from build123d import *

# Parameters (mm, degrees)
BOSS_EXTRUDE1_DEPTH = 14.2875
SKETCH2_R           = 5.9436
BOSS_EXTRUDE2_DEPTH = 0.9906
SKETCH3_R           = 6.35
BOSS_EXTRUDE3_DEPTH = 0.79375
CHAMFER1_SIZE       = 0.254
SKETCH4_R           = 3.175
CUT_EXTRUDE1_DEPTH  = 12.7
BOSS_EXTRUDE4_DEPTH = 43.1165
BOSS_EXTRUDE5_START = 0.9906
SKETCH6_R           = 5.9436
BOSS_EXTRUDE5_DEPTH = 0.9906
BOSS_EXTRUDE6_START = 0.79375
SKETCH7_R           = 6.35
BOSS_EXTRUDE6_DEPTH = 0.79375
CHAMFER2_SIZE       = 0.254


with BuildPart() as part:
    # Sketch1 → Boss-Extrude1 (new, symmetric)
    with BuildSketch(Plane.XY):
        Polygon((7.332348419, 0), (3.666174209, 6.35), (-3.666174209, 6.35), (-7.332348419, 0), (-3.666174209, -6.35), (3.666174209, -6.35), align=None)
    extrude(amount=BOSS_EXTRUDE1_DEPTH, both=True)

    # Sketch2 → Boss-Extrude2 (add)
    with BuildSketch(Plane(origin=(0, 0, -14.2875), x_dir=(-1, 0, 0), z_dir=(0, 0, -1))):
        with Locations(Location((0, 0, 0), (0, 0, 180))):
            Circle(SKETCH2_R)
    extrude(amount=BOSS_EXTRUDE2_DEPTH)

    # Sketch3 → Boss-Extrude3 (add)
    with BuildSketch(Plane(origin=(0, 0, -15.2781), x_dir=(-1, 0, 0), z_dir=(0, 0, -1))):
        Circle(SKETCH3_R)
    extrude(amount=BOSS_EXTRUDE3_DEPTH)

    # Chamfer1
    chamfer1_edges = [part.edges().sort_by_distance(p)[0] for p in [
        (6.35, 0, -16.07185),
    ]]
    chamfer(chamfer1_edges, length=CHAMFER1_SIZE)

    # Sketch4 → Cut-Extrude1 (cut)
    with BuildSketch(Plane(origin=(0, 0, -16.07185), x_dir=(-1, 0, 0), z_dir=(0, 0, -1))):
        Circle(SKETCH4_R)
    extrude(amount=-CUT_EXTRUDE1_DEPTH, mode=Mode.SUBTRACT)

    # Sketch5 → Boss-Extrude4 (add)
    with BuildSketch(Plane.XY.offset(14.2875)):
        Polygon((3.666174209, 6.35), (-3.666174209, 6.35), (-7.332348419, 0), (-3.666174209, -6.35), (3.666174209, -6.35), (7.332348419, 0), align=None)
    extrude(amount=BOSS_EXTRUDE4_DEPTH)

    # Sketch6 → Boss-Extrude5 (add)
    with BuildSketch(Plane.XY.offset(57.404).offset(BOSS_EXTRUDE5_START)):
        Circle(SKETCH6_R)
    extrude(amount=-BOSS_EXTRUDE5_DEPTH)

    # Sketch7 → Boss-Extrude6 (add)
    with BuildSketch(Plane.XY.offset(58.3946).offset(BOSS_EXTRUDE6_START)):
        with Locations(Location((0, 0, 0), (0, 0, 180))):
            Circle(SKETCH7_R)
    extrude(amount=-BOSS_EXTRUDE6_DEPTH)

    # Chamfer2
    chamfer2_edges = [part.edges().sort_by_distance(p)[0] for p in [
        (6.35, 0, 59.18835),
    ]]
    chamfer(chamfer2_edges, length=CHAMFER2_SIZE)


solid = part.part
Design review of the part built by this model. Coordinates are the model's own, in mm. A direction names the side the tool comes from. Round coordinates to 2 decimals unless told otherwise and drop trailing zeros. Write each loop counter-clockwise with the first axis right and the second up, starting at its lowest first coordinate (ties: lowest second). Pieces come first, ordered by that corner, then holes. Notation, with made-up numbers: (-39, 0) - (-10, 0) arc R12 ccw to (-10, 7) - close; hole circle Ø4 at (-17, 85). An arc over 180 degrees is marked (long way). Use a Markdown table: item, result. Add a question column.
1. Wall thickness on probe 1 along Y at (x, z) = (0, -11) (3 decimals); probe 2 along Z at (x, y) = (5, -3.75); probe 3 along X at (y, z) = (2.75, -4.5): over which ranges is each line inside the solid? List them lowest first.
2. For faces 1 (the face through (5.94, -1.38, -14.288)), 2 (the face through (1.38, -6.2, -15.54)), 3 (the face through (-3, -3, -16.072)), list the 3-axis set-ups (+Z, -Z, +X, -X, +Y, -Y) from which the entire face can be reached by the end or side of a thin tool; tool diameter is ignored.
3. Clearance check with flat-ended pins moving along their axes: pin 1 (3 mm diameter, centred on x = 6, z = 23.5, fed in from -Y); pin 2 (4 mm diameter, centred on y = 3.5, z = 9, fed in from +X); pin 3 (4 mm diameter, centred on x = 0, y = 0, fed in from -Z). State where each tip first meets the part, or that it passes through.
4. Mouldability with a two-part tool opening along X and no side actions: class faces 4 (the face through (0, 0, -3.372)), 5 (the face through (-5.474, 3.219, 21.056)), 6 (the face through (-2.93, 5.634, 58.668)) as +X half, -X half, draft (parallel to the pull), parting line (faces both ways), or undercut.
5. We need section B-B (z = 10.5). State the section outline as (x, y) points.
Output:
| question | item | result |
|---|---|---|
| 1 | probe 1 | y = -6.35 to -3.175, 3.175 to 6.35 |
| 1 | probe 2 | z = -15.92 to -15.28, -14.29 to 57.4, 58.39 to 59.03 |
| 1 | probe 3 | x = -5.74 to -1.59, 1.59 to 5.74 |
| 2 | face 1 | none |
| 2 | face 2 | -Z |
| 2 | face 3 | -Z, +X, -X, +Y, -Y |
| 3 | pin 1 | stops at y = -4.91 |
| 3 | pin 2 | stops at x = 6.47 |
| 3 | pin 3 | stops at z = -3.37 |
| 4 | face 4 | undercut |
| 4 | face 5 | -X half |
| 4 | face 6 | parting line |
| 5 | outline | (-7.33, 0) - (-3.67, -6.35) - (3.67, -6.35) - (7.33, 0) - (3.67, 6.35) - (-3.67, 6.35) - close |
